from build123d import *

# Parameters (mm, degrees)
ESQUISSE1_R             = 1.55
BOSS_EXTRU_1_DEPTH      = 8
ENL_V_MAT_EXTRU_1_DEPTH = 4
ESQUISSE3_R             = 4
ENL_V_MAT_EXTRU_2_DEPTH = 8


with BuildPart() as part:
    # Esquisse1 → Boss.-Extru.1 (new body)
    with BuildSketch(Plane.XY):
        with BuildLine():
            Line((-50.035172564, 24.058527132), (-50.035172564, -35.925114983))
            Line((-50.035172564, -35.925114983), (-30.035172564, -35.925114983))
            Line((-30.035172564, -35.925114983), (-30.035172564, -30.046435327))
            ThreePointArc((-30.035172564, -30.046435327), (-30.035172564, -27.925114983), (-27.913852221, -27.925114983))
            Line((-27.913852221, -27.925114983), (17.844379825, -27.925114983))
            ThreePointArc((17.844379825, -27.925114983), (19.965700169, -27.925114983), (19.965700169, -30.046435327))
            Line((19.965700169, -30.046435327), (19.965700169, -35.925114983))
            Line((19.965700169, -35.925114983), (39.964827436, -35.925114983))
            Line((39.964827436, -35.925114983), (39.964827436, 11.93808024))
            ThreePointArc((39.964827436, 11.93808024), (39.957922176, 14.050691679), (42.070406367, 14.074885017))
            Line((42.070406367, 14.074885017), (45.86099397, 14.074885017))
            ThreePointArc((45.86099397, 14.074885017), (47.974344085, 14.04981219), (47.964827436, 11.936334773))
            Line((47.964827436, 11.936334773), (47.964827436, -35.925114983))
            Line((47.964827436, -35.925114983), (249.964827436, -35.925114983))
            Line((249.964827436, -35.925114983), (249.964827436, -5.941472868))
            Line((249.964827436, -5.941472868), (244.087020512, -5.941472868))
            ThreePointArc((244.087020512, -5.941472868), (241.966136804, -5.941909324), (241.964827436, -3.821025976))
            Line((241.964827436, -3.821025976), (241.964827436, 31.937207148))
            ThreePointArc((241.964827436, 31.937207148), (241.964827616, 34.058527312), (244.086147779, 34.058527132))
            Line((244.086147779, 34.058527132), (249.964827436, 34.058527132))
            Line((249.964827436, 34.058527132), (249.964827436, 64.074885017))
            Line((249.964827436, 64.074885017), (64.964827436, 64.074885017))
            Line((64.964827436, 64.074885017), (64.964827436, 46.19620536))
            ThreePointArc((64.964827436, 46.19620536), (64.973452157, 44.066397786), (62.843644031, 44.074885017))
            Line((62.843644031, 44.074885017), (59.087020512, 44.074885017))
            ThreePointArc((59.087020512, 44.074885017), (56.965700528, 44.074011925), (56.964827436, 46.195331909))
            Line((56.964827436, 46.195331909), (56.964827436, 64.074885017))
            Line((56.964827436, 64.074885017), (39.964827436, 64.074885017))
            Line((39.964827436, 64.074885017), (39.964827436, 194.074885017))
            Line((39.964827436, 194.074885017), (22.086147779, 194.074885017))
            ThreePointArc((22.086147779, 194.074885017), (19.964827436, 194.074885017), (19.964827436, 196.19620536))
            Line((19.964827436, 196.19620536), (19.964827436, 202.074885017))
            Line((19.964827436, 202.074885017), (-30.035172564, 202.074885017))
            Line((-30.035172564, 202.074885017), (-30.035172564, 196.19620536))
            ThreePointArc((-30.035172564, 196.19620536), (-30.035172564, 194.074885017), (-32.156492908, 194.074885017))
            Line((-32.156492908, 194.074885017), (-50.035172564, 194.074885017))
            Line((-50.035172564, 194.074885017), (-50.035172564, 24.058527132))
        make_face()
        with Locations((43.965700169, 39.074885017)):
            Circle(ESQUISSE1_R, mode=Mode.SUBTRACT)
        with Locations((-5.034736198, 198.074885017)):
            Circle(ESQUISSE1_R, mode=Mode.SUBTRACT)
        with Locations((245.964827436, -20.925114983)):
            Circle(ESQUISSE1_R, mode=Mode.SUBTRACT)
        with Locations((245.964827481, 49.066706209)):
            Circle(ESQUISSE1_R, mode=Mode.SUBTRACT)
    extrude(amount=BOSS_EXTRU_1_DEPTH)

    # Esquisse2 → Enlèv. mat.-Extru.1 (cut)
    with BuildSketch(Plane.XY.offset(8)):
        with BuildLine():
            Line((60.964827436, 52.074885017), (243.898356115, 52.074885017))
            ThreePointArc((243.898356115, 52.074885017), (245.834400808, 52.256079256), (245.964827436, 54.19620536))
            Line((245.964827436, 54.19620536), (245.964827436, 64.074885017))
            Line((245.964827436, 64.074885017), (60.964827436, 64.074885017))
            Line((60.964827436, 64.074885017), (60.964827436, 52.074885017))
        make_face()
    extrude(amount=-ENL_V_MAT_EXTRU_1_DEPTH, mode=Mode.SUBTRACT)

    # Esquisse3 → Enlèv. mat.-Extru.2 (cut)
    with BuildSketch(Plane.XY.offset(8)):
        with Locations((-30.035172564, -15.925114983)):
            Circle(ESQUISSE3_R)
    extrude(amount=-ENL_V_MAT_EXTRU_2_DEPTH, mode=Mode.SUBTRACT)


solid = part.part
Geometry check sheet. Reference: the model listing, model coordinates, mm. A direction names the side the tool comes from. Give positions to 0.01 mm unless a question says otherwise; leave off trailing zeros. Order: outer loops, then holes, each group sorted by start corner. A loop starts at its lowest first (then second) coordinate and runs counter-clockwise, first axis right, second up. Notation, with made-up numbers: (86.25, 0.25) - (100.25, 0.25) arc R9 cw to (100.25, 11.25) - close; hole circle Ø10 at (29.25, 51). An arc over 180 degrees is marked (long way). Answer as a JSON object with one key per item and string values.
(1) Tool access check on faces 1 (the flat face through (64.965, 53, 3)), 2 (the flat face through (-41, 194.075, 4)), 3 (the flat face through (-5, -27.925, 4)), 4 (the flat face through (39.965, 128, 4)). Record the directions out of +Z, -Z, +X, -X, +Y, -Y that give a thin tool (end or side, any length) a straight path to the whole face; none if there is none.
Report:
{"face 1": "+Z, -Z, +Y", "face 2": "+Z, -Z, -X, +Y", "face 3": "+Z, -Z, -Y", "face 4": "+Z, -Z, +X, +Y"}
(2) Draft check along Y on faces 5 (the flat face through (-40, -35.925, 4)), 6 (the flat face through (31, 194.075, 4)), 7 (the flat face through (247, -5.941, 4)). Enter one of: released by +Y, released by -Y, zero draft, split by the parting line, or undercut.
Report:
{"face 5": "released by -Y", "face 6": "released by +Y", "face 7": "undercut"}
(3) Cross-section at A-A (y = 23.5). Record the cut outline in (x, z), then the cut area to 3 significant figures.
Report:
{"outline": "(-50.04, 0) - (241.96, 0) - (241.96, 8) - (-50.04, 8) - close", "area": "2,340 mm^2"}
(4) Cross-section at D-D (y = 113). Record the cut outline in (x, z).
Report:
{"outline": "(-50.04, 0) - (39.96, 0) - (39.96, 8) - (-50.04, 8) - close"}
(5) Depth check by flat-ended pin: pin 1 Ø2 at (x, y) = (-15, 46.5) entering from -Z; pin 2 Ø2.5 at (y, z) = (147.5, 3.5) entering from +X; pin 3 Ø1.1 at (x, z) = (61.5, 4.5) entering from +Y; pin 4 Ø4.5 at (x, z) = (114, 5.5) entering from +Y. Enter the tip coordinate at first touch or a pass-through.
Report:
{"pin 1": "z = 0", "pin 2": "x = 39.96", "pin 3": "y = 44.07", "pin 4": "y = 64.07"}
(6) Cross-section at C-C (z = 2.25). State how many separate pieces and enclosed holes the cut face has, then the cut area to 3 significant figures.
Report:
{"separate pieces": "1", "enclosed holes": "5", "area": "40,700 mm^2"}
(7) Cross-section at B-B (x = 108.5). Record the cut outline in (y, z), then the cut area to 3 significant figures.
Report:
{"outline": "(-35.93, 0) - (64.07, 0) - (64.07, 4) - (52.07, 4) - (52.07, 8) - (-35.93, 8) - close", "area": "752 mm^2"}
(8) Material ranges on line 1 (X direction, y = 8.5, z = 3); line 2 (X direction, y = -9, z = 5.5); line 3 (Y direction, x = 92.5, z = 2), recorded low to high.
Report:
{"line 1": "-50.04 to 39.96, 47.96 to 241.96", "line 2": "-50.04 to 39.96, 47.96 to 249.96", "line 3": "-35.93 to 64.07"}
